Could you check a few things on this model? Use its own coordinates, in mm. A direction names the side the tool comes from. Coordinates: 2 decimals unless noted, no trailing zeros. Loops run counter-clockwise (first coordinate to the right, second up) from the corner with the lowest first, then second, coordinate; pieces in that order, holes last.
1) Imagine slicing it at A-A on y = 0. Please give me the cut outline in (x, z), plus the area to 3 significant figures.
2) Imagine slicing it at C-C on y = 4.75. Please give me the cut outline in (x, z), plus the area to 3 significant figures.
3) If I drill on line 1 along Y through (x, z) = (2.75, -4.75); line 2 along Y through (x, z) = (2.75, 0.25); line 3 along Y through (x, z) = (0.7, -6.25), over which ranges is the centre line in solid material (lowest first)?
4) Imagine slicing it at B-B on z = -0.25. Please give me the cut outline in (x, y).
5) Will these pins go through, and if not, where does the flat tip stop? P1, Ø1, axis at x = 3, z = -4, coming from the -Y side; P2, Ø1.5, axis at x = 3.5, z = -0.5, coming from the +Y side; P3, Ø6, axis at y = -0.5, z = -2, coming from the +X side; P4, Ø2.5, axis at x = 3, y = 2, coming from the -Z side.
6) For faces 4 (the face through (2.465, -3.868, 6.714)), 5 (the face through (2.46, 6.28, 6.33)), 6 (the face through (2.46, -5.17, -7.3)), which set-ups out of +Z, -Z, +X, -X, +Y, -Y let a thin tool reach every point of the face, with its end or its side?
7) Thinking about a two-plate mould opening in Z: for faces 1 (the face through (2.465, -8.064, -3.8)), 2 (the face through (2.46, -2.34, 8.6)), 3 (the face through (2.46, -2.36, -8.63)), which applies, released by +Z, released by -Z, zero draft, split by the parting line, or undercut?
```python
from build123d import *

# Parameters (mm, degrees)
BASPROSKE_W        = 5
BASPROSKE_H        = 10
TOOTHCUT_DEPTH     = 16
TEETHCUTS_COUNT    = 18
TEETHCUTS_ANGLE    = 340
BORSKE_R           = 2.5
BORE_DEPTH         = 50.0000508
SKETCH1_W          = 8
SKETCH1_H          = 8
CUT_EXTRUDE1_DEPTH = 15.925454152


with BuildPart() as part:
    # BasProSke → Base-Revolve (revolve)
    with BuildSketch(Plane(origin=(0, 0, 0), x_dir=(1, 0, 0), z_dir=(0, 1, 0)), mode=Mode.PRIVATE) as base_revolve_sk:
        with Locations((2.5, 5)):
            Rectangle(BASPROSKE_W, BASPROSKE_H)
    revolve(base_revolve_sk.sketch.rotate(Axis((-10, 0, 0), (1, 0, 0)), 180), axis=Axis((-10, 0, 0), (1, 0, 0)))

    # TooCutSke → ToothCut (cut, through all)
    with BuildSketch(Plane(origin=(0, 0, 0), x_dir=(0, 0, -1), z_dir=(1, 0, 0))):
        with BuildLine():
            ThreePointArc((0.510641536, 7.732156635), (0, 7.749), (-0.510641536, 7.732156635))
            ThreePointArc((-0.510641536, 7.732156635), (-0.82619259, 8.907320741), (-1.515208602, 9.910236529))
            ThreePointArc((-1.515208602, 9.910236529), (0, 10.0254), (1.515208602, 9.910236529))
            ThreePointArc((1.515208602, 9.910236529), (0.82619259, 8.907320741), (0.510641536, 7.732156635))
        make_face()
    toothcut = extrude(amount=TOOTHCUT_DEPTH, mode=Mode.SUBTRACT)

    # TeethCuts: ToothCut ×18 about axis
    teethcuts_axis = Axis((-10, 0, 0), (1, 0, 0))
    for i in range(1, TEETHCUTS_COUNT):
        add(toothcut.rotate(teethcuts_axis, i * TEETHCUTS_ANGLE / (TEETHCUTS_COUNT - 1)), mode=Mode.SUBTRACT)

    # BorSke → Bore (cut, symmetric)
    with BuildSketch(Plane(origin=(0, 0, 0), x_dir=(0, 0, -1), z_dir=(1, 0, 0))):
        with Locations(Location((0, 0, 0), (0, 0, 180))):
            Circle(BORSKE_R)
    extrude(amount=BORE_DEPTH, both=True, mode=Mode.SUBTRACT)

    # Sketch1 → Cut-Extrude1 (cut, through all)
    with BuildSketch(Plane(origin=(5, 0, 0), x_dir=(0, 0, -1), z_dir=(1, 0, 0))):
        Rectangle(SKETCH1_W, SKETCH1_H)
    extrude(amount=-CUT_EXTRUDE1_DEPTH, mode=Mode.SUBTRACT)


solid = part.part
```
Filled in:
1. outline: (0, -10) - (5, -10) - (5, -4) - (0, -4) - close; (0, 4) - (5, 4) - (5, 10) - (0, 10) - close
1. area: 60.0 mm2
2. outline: (0, -6.95) - (5, -6.95) - (5, 6.95) - (0, 6.95) - close
2. area: 69.5 mm2
3. line 1: y = -8.76 to -6.52, -6.12 to 6.12, 6.52 to 8.76
3. line 2: y = -7.74 to -4, 4 to 7.74
3. line 3: y = -6.24 to 6.24
4. outline: (0, -7.74) - (5, -7.74) - (5, -4) - (0, -4) - close; (0, 4) - (5, 4) - (5, 7.74) - (0, 7.74) - close
5. P1: stops at y = -8.62
5. P2: stops at y = 9.61
5. P3: stops at x = 5
5. P4: stops at z = -9.48
6. face 4: +X, -X
6. face 5: +X, -X, +Y
6. face 6: -Z, +X, -X
7. face 1: undercut
7. face 2: released by +Z
7. face 3: released by -Z
